The figure shows three views and two pictorial views of one solid part (mm, origin at its lowest corner). Answer the questions. A direction names the side the tool comes from. Round coordinates to 2 decimals unless told otherwise and drop trailing zeros. Write each loop counter-clockwise with the first axis right and the second up, starting at its lowest first coordinate (ties: lowest second). Pieces come first, ordered by that corner, then holes. Notation, with made-up numbers: M 86,-8.75 L 139,-8.75 A23 ccw 139,18.25 Z; hole C 44,16 d9. An arc over 180 degrees is marked long. One line per item, written item: value. Start each with the question number.
Q1. Consider probe 1 along Z at (x, y) = (15.5, 2); probe 2 along Z at (x, y) = (14, 0.7) (1 decimal); probe 3 along X at (y, z) = (1.05, 3.75). Determine where each line is inside the solid, lowest interval first.
Q2. Find section A-A (x = 10). Write down the section's boundary in (y, z) (1 decimal).
Q3. A tool of negligible diameter and unlimited length cuts with its end or side. For the marked faces 1, 2, 3, 4 and 5, from which of +Z, -Z, +X, -X, +Y, -Y can it reach the whole face along a straight path? Write none if from no direction.
Q4. Find section C-C (x = 14.75). Write down the section's boundary in (y, z) (1 decimal).
Q5. Find section D-D (x = 20.5). Write down the section's boundary in (y, z) (1 decimal).
Q6. Given pin 1 Ø1.6 at (y, z) = (2.5, 2.5) entering from +X; pin 2 Ø1.6 at (y, z) = (2, 3) entering from -X, each flat-ended and moving along its own axis, determine where each tip first touches the part or whether it passes through.
Q7. Find section B-B (z = 1.25). Write down the section's boundary in (x, y) (1 decimal).
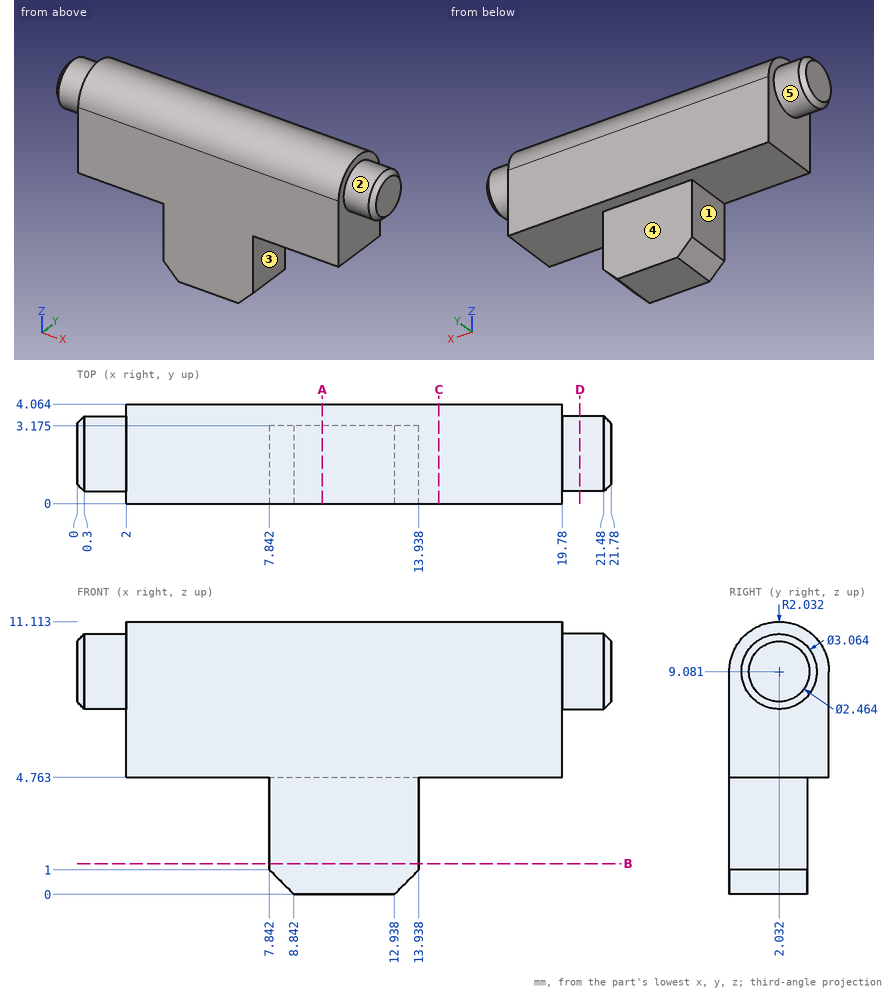
The answers:
1. probe 1: 4.76 to 11.11
1. probe 2: 4.8 to 10.6
1. probe 3: 7.84 to 13.94
2. outline: M 0,0 L 3.2,0 L 3.2,4.8 L 4.1,4.8 L 4.1,9.1 A2 ccw 0,9.1 Z
3. face 1: -Z, -X, +Y, -Y
3. face 2: +X
3. face 3: -Z, +X, +Y, -Y
3. face 4: -Z, +X, -X, +Y
3. face 5: -X
4. outline: M 0,4.8 L 4.1,4.8 L 4.1,9.1 A2 ccw 0,9.1 Z
5. outline: C 2,9.1 d3.1
6. pin 1: x = 13.94
6. pin 2: x = 7.84
7. outline: M 7.8,0 L 13.9,0 L 13.9,3.2 L 7.8,3.2 Z
